Source: CAD feature listing. Evaluate the final solid. Frame: model axes, mm. A direction names the side the tool comes from. Coordinates: 2 decimals unless noted, no trailing zeros. Loops run counter-clockwise (first coordinate to the right, second up) from the corner with the lowest first, then second, coordinate; pieces in that order, holes last.
```python
from build123d import *

# Parameters (mm, degrees)
F1_DEPTH = 5
F2_DEPTH = 200
F5_DEPTH = 5


with BuildPart() as f1:
    # F0 (on Front) → F1 (new body)
    with BuildSketch(Plane.XZ):
        Polygon((-100, -14.5512985522), (-100, 0), (-100, 100), (-105, 105), (-105, 200), (-195, 200), (-195, 80.4487014478), align=None)
        Polygon((-100, -21.6223663641), (-100, -14.5512985522), (-195, 80.4487014478), (-195, 200), (-200, 200), (-200, 78.3776336359), align=None)
        Polygon((-105, 105), (-100, 100), (-100, 200), (-105, 200), align=None)
    extrude(amount=-F1_DEPTH)

    # F0 (on Front) → F2 (join)
    with BuildSketch(Plane.XZ):
        Polygon((-100, -21.6223663641), (-100, -14.5512985522), (-195, 80.4487014478), (-195, 200), (-200, 200), (-200, 78.3776336359), align=None)
        Polygon((-105, 105), (-100, 100), (-100, 200), (-105, 200), align=None)
    extrude(amount=F2_DEPTH)

    # F4 (on offset) → F5 (join)
    with BuildSketch(Plane.XZ.offset(200)):
        Polygon((-100, -21.7671551462), (-100, 200), (-200, 200), (-200, 77.8633803129), align=None)
    extrude(amount=F5_DEPTH)


solid = f1.part
```
Q1. Material intervals for line 1 along X through (y, z) = (-18, 170); line 2 along Y through (x, z) = (-155, 78.5); line 3 along X through (y, z) = (-126.5, 84), sorted ascending.
Q2. Section query B-B on z = 124. Return the cut outline in (x, y).
Q3. Section query C-C on x = -159.5. Return the cut outline in (y, z), then the cut area to 3 significant figures.
Q4. Section query A-A on y = -113.5. Return the cut outline in (x, z).
Q5. Section query D-D on z = 69. Return the cut outline in (x, y).
Q6. Draft query along X for faces 4 (the flat face through (-100, -99, 161)), 5 (the flat face through (-195, -99, 139)), 6 (the flat face through (-102, -100, 200)). Return one class per face: released by +X, released by -X, zero draft, split by the parting line, or undercut.
Q7. First-contact query: pin 1 Ø1.5 at (x, y) = (-152.5, -34) entering from -Z; pin 2 Ø10 at (x, y) = (-115, -158) entering from -Z. Flat tips, straight axial feed; report the tip coordinate or a pass-through.
Q8. Reachability of faces 1 (the flat face through (-105, -99, 153)), 2 (the flat face through (-150.7, -96.06, 29.08)), 3 (the flat face through (-103, -99, 103)) from +Z, -Z, +X, -X, +Y, -Y: full face, straight path, thin tool, end or side. Return the list, or none.
Resolved:
1. line 1: x = -200 to -195, -105 to -100
1. line 2: y = -205 to -200, 0 to 5
1. line 3: x = -200 to -195
2. outline: (-200, -205) - (-100, -205) - (-100, 5) - (-200, 5) - close; hole (-195, -200) - (-105, -200) - (-105, 0) - (-195, 0) - close
3. outline: (-205, 37.51) - (-200, 37.51) - (-200, 37.88) - (5, 37.88) - (5, 200) - (0, 200) - (0, 44.95) - (-200, 44.95) - (-200, 200) - (-205, 200) - close
3. area: 3,040 mm2
4. outline: (-200, 78.38) - (-100, -21.62) - (-100, -14.55) - (-195, 80.45) - (-195, 200) - (-200, 200) - close; (-105, 105) - (-100, 100) - (-100, 200) - (-105, 200) - close
5. outline: (-191.1, -205) - (-100, -205) - (-100, -200) - (-183.55, -200) - (-183.55, 0) - (-100, 0) - (-100, 5) - (-190.62, 5) - (-190.62, -200) - (-191.1, -200) - close
6. face 4: released by +X
6. face 5: undercut
6. face 6: zero draft
7. pin 1: stops at z = 30.13
7. pin 2: stops at z = -11.62
8. face 1: +Z
8. face 2: -Z, -X, +Y
8. face 3: none
